Read the model definition and answer for the solid it produces. Units are mm, in the model's axes. Round coordinates to 2 decimals unless told otherwise and drop trailing zeros. Loops run counter-clockwise (first coordinate to the right, second up) from the corner with the lowest first, then second, coordinate; pieces in that order, holes last. Notation, with made-up numbers: (66.5, 78) -> (102.5, 78) arc R16 ccw to (102.5, 100) -> close; hole circle Ø5 at (-25.75, -5.75). An arc over 180 degrees is marked (long way). Put each result on its own line as item: value.
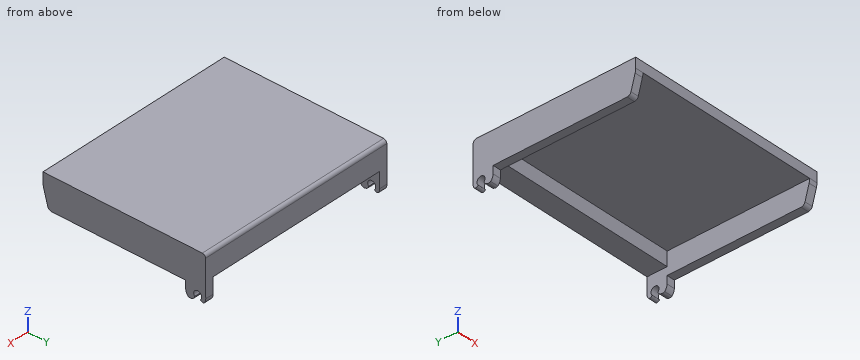
from build123d import *

# Parameters (mm, degrees)
BOSS_EXTRUDE1_DEPTH = 50
FILLET5_R           = 2
SKETCH5_W           = 46
SKETCH5_H           = 5.5
CUT_EXTRUDE1_DEPTH  = 35.5
SKETCH6_R           = 1
CUT_EXTRUDE2_DEPTH  = 50
FILLET8_R           = 2
CUT_EXTRUDE3_DEPTH  = 50
CUT_EXTRUDE4_REACH  = 73.453
CUT_EXTRUDE4_START  = -6
SKETCH9_W           = 46
SKETCH9_H           = 5.08594255


with BuildPart() as part:
    # Sketch1 → Boss-Extrude1 (new body)
    with BuildSketch(Plane(origin=(0, 0, 0), x_dir=(0, 0, -1), z_dir=(1, 0, 0))):
        with BuildLine():
            Line((-3.886543853, 40.629191905), (-3.858449328, 35.629270836))
            Line((-3.858449328, 35.629270836), (-7.758387762, 35.607357106))
            Line((-7.758387762, 35.607357106), (-7.570756078, 2.214957203))
            ThreePointArc((-7.570756078, 2.214957203), (-7.773978903, 1.605044256), (-8.306497887, 1.244882))
            Line((-8.306497887, 1.244882), (-12.050945383, 0.218975681))
            ThreePointArc((-12.050945383, 0.218975681), (-12.563535137, 0.11401769), (-13.085439382, 0.076864019))
            Line((-13.085439382, 0.076864019), (-15.558790346, 0.062966276))
            Line((-15.558790346, 0.062966276), (-15.781860873, 39.762339565))
            ThreePointArc((-15.781860873, 39.762339565), (-15.55072853, 40.329332651), (-14.986368626, 40.56682206))
            Line((-14.986368626, 40.56682206), (-3.886543853, 40.629191905))
        make_face()
    extrude(amount=-BOSS_EXTRUDE1_DEPTH)

    # Fillet5
    fillet5_edges = [part.edges().sort_by_distance(p)[0] for p in [
        (-25, 35.629270836, 3.858449328),
    ]]
    fillet(fillet5_edges, radius=FILLET5_R)

    # Sketch5 → Cut-Extrude1 (cut)
    with BuildSketch(Plane(origin=(0, 0.150386272, 0.00084502), x_dir=(1, 0, 0), z_dir=(0, -0.9999842138288617, -0.005618904971023238))):
        with Locations((-25, 10.308190931)):
            Rectangle(SKETCH5_W, SKETCH5_H)
    extrude(amount=-CUT_EXTRUDE1_DEPTH, mode=Mode.SUBTRACT)

    # Sketch6 → Cut-Extrude2 (cut)
    with BuildSketch(Plane(origin=(0, 0, 0), x_dir=(0, 0, -1), z_dir=(1, 0, 0))):
        with Locations((-5.775276049, 38.618547558)):
            Circle(SKETCH6_R)
    extrude(amount=-CUT_EXTRUDE2_DEPTH, mode=Mode.SUBTRACT)

    # Fillet8
    fillet8_edges = [part.edges().sort_by_distance(p)[0] for p in [
        (-25, 40.629191905, 3.886543853),
    ]]
    fillet(fillet8_edges, radius=FILLET8_R)

    # Sketch7 → Cut-Extrude3 (cut)
    with BuildSketch(Plane(origin=(0, 0, 0), x_dir=(0, 0, -1), z_dir=(1, 0, 0))):
        with BuildLine():
            Line((-5.546917351, 39.592124625), (-5.546917351, 37.644970491))
            add(Edge.make_bspline(
                [(-5.546917351, 37.644970491), (-4.707853676, 38.427857511), (-3.932802052, 36.795264926), (-4.447517997, 36.211756548)],
                knots=[0, 0, 0, 0, 1, 1, 1, 1], degree=3))
            Line((-4.447517997, 36.211756548), (-3.72986133, 36.211756548))
            Line((-3.72986133, 36.211756548), (-3.72986133, 40.421981197))
            Line((-3.72986133, 40.421981197), (-5.011793069, 40.421981197))
            add(Edge.make_bspline(
                [(-5.272048409, 39.482701446), (-5.081010169, 39.321292536), (-4.954269224, 39.348440279), (-4.587478606, 39.771100718), (-4.694245253, 40.267694009), (-5.011793069, 40.421981197)],
                knots=[0, 0, 0, 0, 0.130864933, 0.344471665, 1, 1, 1, 1], degree=3))
            add(Edge.make_bspline(
                [(-5.546917351, 39.592124625), (-5.444164643, 39.566706147), (-5.272048409, 39.482701446)],
                knots=[0, 0, 0, 1, 1, 1], degree=2))
        make_face()
    extrude(amount=-CUT_EXTRUDE3_DEPTH, mode=Mode.SUBTRACT)

    # Sketch9 → Cut-Extrude4 (cut, up to next)
    with BuildSketch(Plane(origin=(0, -0.087419996, 15.557945326), x_dir=(1, 0, 0), z_dir=(0, -0.00561890497102722, 0.9999842138288618)).offset(CUT_EXTRUDE4_START), mode=Mode.PRIVATE) as cut_extrude4_sk1:
        with Locations((-25, 38.193359921)):
            Rectangle(SKETCH9_W, SKETCH9_H)
    cut_extrude4_tool1 = extrude(cut_extrude4_sk1.sketch, amount=-CUT_EXTRUDE4_REACH, mode=Mode.PRIVATE) & part.part
    add(cut_extrude4_tool1.solids().sort_by_distance((-25, 38.13905, 9.772645))[0], mode=Mode.SUBTRACT)


solid = part.part
Item 1: The part is cut by section B-B (z = 11). Determine the outline of the cut face in (x, y).
Derived:
outline: (-50, 0.51) -> (-48, 0.51) -> (-48, 35.59) -> (-2, 35.59) -> (-2, 0.51) -> (0, 0.51) -> (0, 40.59) -> (-50, 40.59) -> close
Item 2: Find the intervals of material crossed by line 1 along X through (y, z) = (3, 10.5); line 2 along Y through (x, z) = (-48, 14.5); line 3 along Y through (x, z) = (-41, 12.25), in increasing order.
Derived:
line 1: x = -50 to -48, -2 to 0
line 2: y = 0.07 to 40.57
line 3: y = 35.58 to 40.58
Item 3: Flat-ended cylindrical pins translate along their axes: pin 1 Ø1.8 at (y, z) = (38.62, 5.78) entering from -X; pin 2 Ø2 at (x, y) = (-15.5, 4.5) entering from -Z; pin 3 Ø4 at (x, z) = (-6.5, 10) entering from +Y; pin 4 Ø12 at (x, y) = (-44, 13) entering from -Z. Find the tip coordinate at first contact, or state that the pin passes through.
Derived:
pin 1: passes through
pin 2: stops at z = 13.08
pin 3: stops at y = 40.6
pin 4: stops at z = 7.61
